Print and shaded views of the part. All mm, measured from the part's lowest x, y and z. A direction names the side the tool comes from. Give positions to 0.01 mm unless a question says otherwise; leave off trailing zeros. Loops run counter-clockwise (first coordinate to the right, second up) from the corner with the lowest first, then second, coordinate; pieces in that order, holes last. Notation, with made-up numbers: M 77.5,7.25 L 120.5,7.25 A27 cw 120.5,41.25 Z; hole C 0,68.5 d4. An arc over 180 degrees is marked long. Answer as CSV lines item,"result".
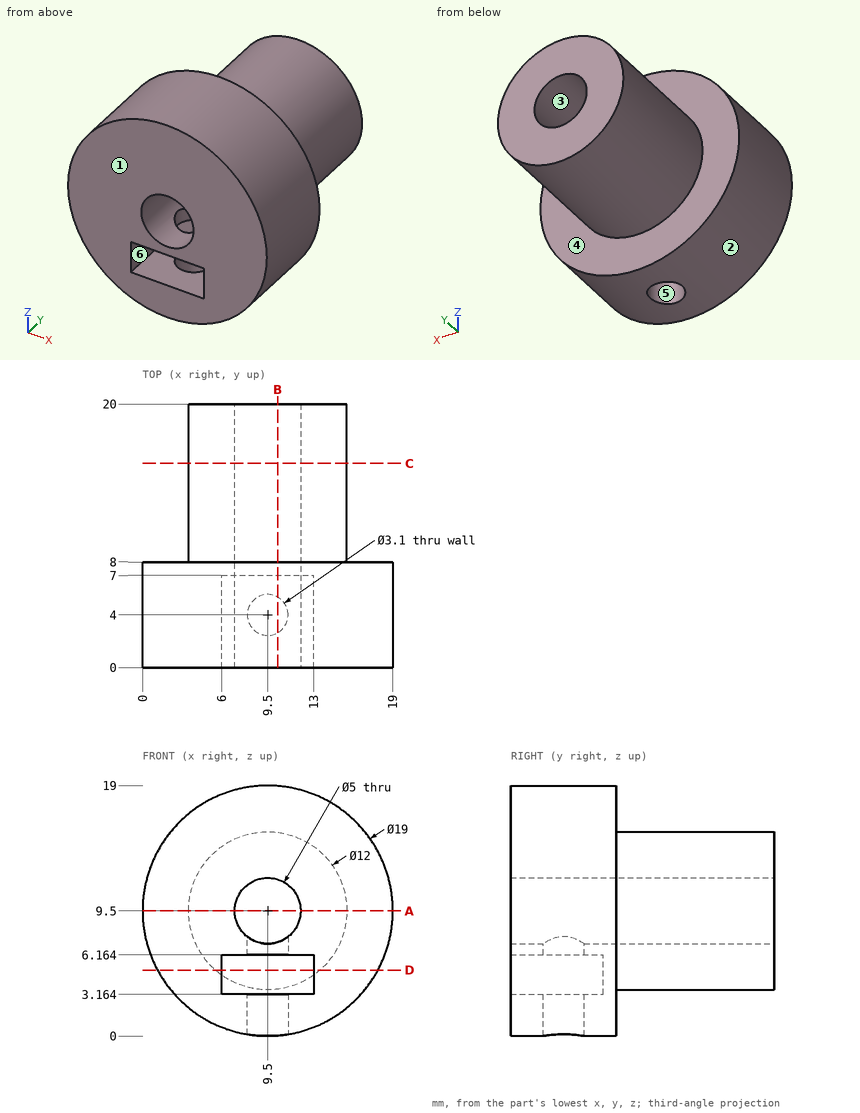
Q1. Mould opens along Z. For the marked faces 1, 2 and 3 say: released by +Z, released by -Z, zero draft, split by the parting line, or undercut.
Solution:
face 1,"zero draft"
face 2,"split by the parting line"
face 3,"undercut"
Q2. Cut at B-B (x = 10.25). Write the cut outline in (y, z) (1 decimal), and give its area (3 significant figures).
Solution:
outline,"M 0,0 L 2.6,0 L 2.6,3.2 L 0,3.2 Z; M 0,6.2 L 2.6,6.2 L 2.6,7.1 L 0,7.1 Z; M 0,11.9 L 20,11.9 L 20,15.5 L 8,15.5 L 8,19 L 0,19 Z; M 5.4,0 L 8,0 L 8,3.5 L 20,3.5 L 20,7.1 L 5.4,7.1 L 5.4,6.2 L 7,6.2 L 7,3.2 L 5.4,3.2 Z"
area,"167 mm²"
Q3. Which spindle directions (+Z, -Z, +X, -X, +Y, -Y) get a long thin tool onto all of the face, cutting with end or side? Do the marked faces 4, 5 and 6. Say none if no direction does.
Solution:
face 4,"+Y"
face 5,"-Z"
face 6,"-Y"
Q4. Cut at D-D (z = 5). Write the cut outline in (x, y), and give its area (3 significant figures).
Solution:
outline,"M 1.13,0 L 6,0 L 6,7 L 13,7 L 13,0 L 17.87,0 L 17.87,8 L 13.47,8 L 13.47,20 L 5.53,20 L 5.53,8 L 1.13,8 Z"
area,"180 mm²"
Q5. Cut at C-C (y = 15.5). Write the cut outline in (x, z).
Solution:
outline,"C 9.5,9.5 d12; hole C 9.5,9.5 d5"
Q6. Cut at A-A (z = 9.5). Write the cut outline in (x, y), and give its area (3 significant figures).
Solution:
outline,"M 0,0 L 7,0 L 7,20 L 3.5,20 L 3.5,8 L 0,8 Z; M 12,0 L 19,0 L 19,8 L 15.5,8 L 15.5,20 L 12,20 Z"
area,"196 mm²"
Q7. Wall check: line 1 (Z direction, x = 9.5, y = 6.5); line 2 (Z direction, x = 9.5, y = 15); line 3 (Y direction, x = 9.5, z = 1.1). Give the ranges that are in metal, low to high. Write a range as [from, to].
Solution:
line 1,"z = [0, 3.16], [6.16, 7], [12, 19]"
line 2,"z = [3.5, 7], [12, 15.5]"
line 3,"y = [0, 2.45], [5.55, 8]"
Q8. Pin check, flat tips, straight feed: P1, Ø1.5, axis at x = 8, y = 8, coming from the -Z side; P2, Ø4, axis at x = 13.5, y = 5, coming from the +Z side; P3, Ø3.5, axis at y = 3.5, z = 5, coming from the +X side. Stop position of each tip, or through.
Solution:
P1,"stops at z = 0.03"
P2,"stops at z = 18.79"
P3,"stops at x = 18.59"
